The listing builds one solid part. Answer for the finished solid, in the listing's coordinates (mm). Face numbers are marked on the shaded views. A direction names the side the tool comes from. Give positions to 0.01 mm unless a question says otherwise; leave off trailing zeros. Write each loop counter-clockwise with the first axis right and the second up, starting at its lowest first coordinate (ties: lowest second). Pieces come first, ordered by that corner, then holes. Notation, with made-up numbers: (-12, -2) - (19, -2) arc R14 ccw to (19, 15) - close; hole circle Ø9 at (60, -27.75). An arc over 180 degrees is marked (long way). One line per item, written item: value. Start each with the question number.
from build123d import *

# Parameters (mm, degrees)
SALIENTE_EXTRUIR1_DEPTH = 10
CROQUIS2_R              = 5
SALIENTE_EXTRUIR4_DEPTH = 10
SALIENTE_EXTRUIR5_START = 10
CROQUIS4_R              = 5
SALIENTE_EXTRUIR5_DEPTH = 10
SALIENTE_EXTRUIR7_START = -10
SALIENTE_EXTRUIR7_DEPTH = 10
CROQUIS8_R              = 5
SALIENTE_EXTRUIR8_DEPTH = 5
SALIENTE_EXTRUIR9_START = 5
CROQUIS10_R             = 5
SALIENTE_EXTRUIR9_DEPTH = 5


with BuildPart() as part:
    # Croquis1 → Saliente-Extruir1 (new body)
    with BuildSketch(Plane.XY):
        Polygon((0, 0), (40, 0), (40, -65), (0, -65), (0, -55), (30, -55), (30, -10), (0, -10), align=None)
    extrude(amount=SALIENTE_EXTRUIR1_DEPTH)

    # Croquis2 → Saliente-Extruir4 (add)
    with BuildSketch(Plane.XZ.offset(10)):
        with Locations(Location((5, 5, 0), (0, 0, 180))):
            Circle(CROQUIS2_R)
    extrude(amount=SALIENTE_EXTRUIR4_DEPTH)

    # Croquis4 → Saliente-Extruir5 (add)
    with BuildSketch(Plane(origin=(0, -55, 0), x_dir=(1, 0, 0), z_dir=(0, 1, 0)).offset(SALIENTE_EXTRUIR5_START)):
        with Locations(Location((5, -5, 0), (0, 0, 180))):
            Circle(CROQUIS4_R)
    extrude(amount=-SALIENTE_EXTRUIR5_DEPTH)

    # Croquis7 → Saliente-Extruir7 (add)
    with BuildSketch(Plane(origin=(0, 0, 0), x_dir=(1, 0, 0), z_dir=(0, 1, 0)).offset(SALIENTE_EXTRUIR7_START)):
        Polygon((30, -5.857864376), (103.639610307, 67.781745931), (110.710678119, 60.710678119), (40, -10), (30, -10), align=None)
    saliente_extruir7 = extrude(amount=-SALIENTE_EXTRUIR7_DEPTH)

    # Simetría1: Saliente-Extruir7 across plane
    add(saliente_extruir7.mirror(Plane.ZX.offset(-32.5)))

    # Croquis8 → Saliente-Extruir8 (add)
    with BuildSketch(Plane.XZ.offset(20)):
        with Locations(Location((103.639610307, -60.710678119, 0), (0, 0, 45))):
            Circle(CROQUIS8_R)
    extrude(amount=SALIENTE_EXTRUIR8_DEPTH)

    # Croquis10 → Saliente-Extruir9 (add)
    with BuildSketch(Plane(origin=(0, -45, 0), x_dir=(1, 0, 0), z_dir=(0, 1, 0)).offset(SALIENTE_EXTRUIR9_START)):
        with Locations(Location((103.639610307, 60.710678119, 0), (0, 0, 315))):
            Circle(CROQUIS10_R)
    extrude(amount=-SALIENTE_EXTRUIR9_DEPTH)


solid = part.part
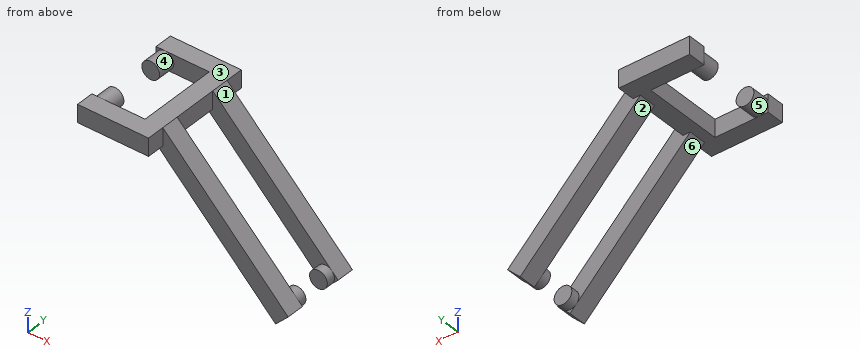
Item 1: Each of these flat-tipped pins is pushed along its axis until it touches: pin 1 Ø8 at (x, z) = (102.5, -62) entering from +Y; pin 2 Ø21.5 at (x, z) = (73.5, -40) entering from -Y; pin 3 Ø8 at (y, z) = (-18.5, -43.5) entering from -X. Where does it stop, or does it pass through?
Item 2: Find section C-C on z = -23.5. Determine the outline of the cut face in (x, y).
Item 3: Find section A-A on y = -11.5. Determine the outline of the cut face in (x, z).
Item 4: The mould has two halves that part along X. Classify the marked faces 1, 2, 3 and 4: +X half, -X half, draft (parallel to the pull), parting line (faces both ways), or undercut.
Item 5: Find section B-B on x = 44. Determine the outline of the cut face in (y, z).
Item 6: Straight lines are drawn through the part: line 1 along Z through (x, y) = (21, -9.5); line 2 along Z through (x, y) = (61, -51); line 3 along X through (y, z) = (-53.5, -37.5). For each, find the intervals that lie inside material, in ascending order.
Item 7: For the marked faces 5 and 6, determine the directions among +Z, -Z, +X, -X, +Y, -Y from which every point of the face is accessible in a straight line to the end or side of a thin tool.
Values:
1. pin 1: y = -10
1. pin 2: y = -55
1. pin 3: x = 75.36
2. outline: (59.36, -55) - (73.5, -55) - (73.5, -45) - (59.36, -45) - close; (59.36, -20) - (73.5, -20) - (73.5, -10) - (59.36, -10) - close
3. outline: circle Ø10 at (5, 5); (30, 0) - (35.86, 0) - (103.64, -67.78) - (110.71, -60.71) - (40, 10) - (30, 10) - close
4. face 1: +X half
4. face 2: -X half
4. face 3: draft
4. face 4: undercut
5. outline: (-55, -8.14) - (-45, -8.14) - (-45, 6) - (-55, 6) - close; (-20, -8.14) - (-10, -8.14) - (-10, 6) - (-20, 6) - close
6. line 1: 0 to 10
6. line 2: -25.14 to -11
6. line 3: 73.36 to 87.5
7. face 5: none
7. face 6: -Z, -X, +Y, -Y
